The drawing under review shows one solid part. Ordinate dimensions are in mm from its lowest x, y, z. A direction names the side the tool comes from. Round coordinates to 2 decimals unless told otherwise and drop trailing zeros. Write each loop counter-clockwise with the first axis right and the second up, starting at its lowest first coordinate (ties: lowest second). Pieces come first, ordered by that corner, then holes. Notation, with made-up numbers: (-2, 51.5) -> (5, 51.5) arc R20 cw to (5, 72.5) -> close; hole circle Ø8 at (56.25, -12.5). An arc over 180 degrees is marked (long way). Answer in a Markdown table with one row per item. Add a question column.
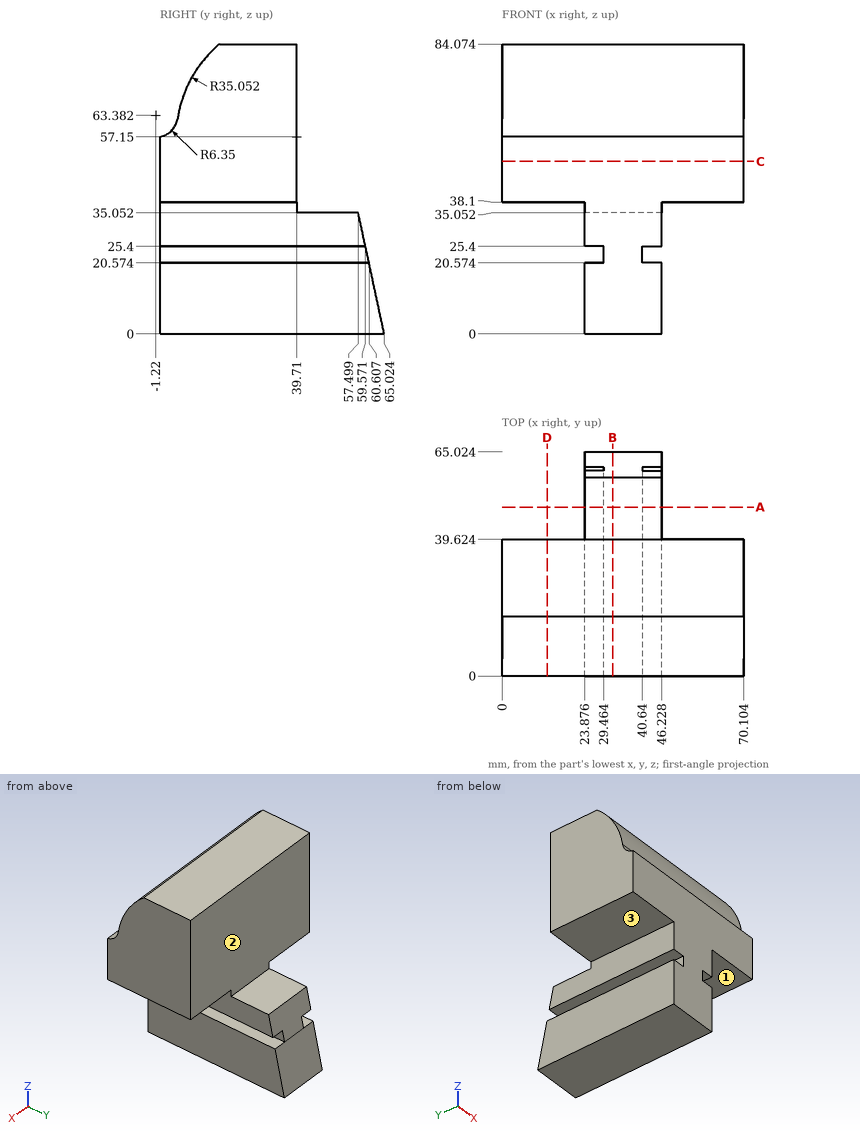
1. Add section C-C on z = 50. Write out the cut boundary in (x, y), plus the area to 3 significant figures.
2. Add section A-A on y = 49. Write out the cut boundary in (x, z).
3. For L1, parallel to Z at x = 41, y = 40.5; L2, parallel to Y at x = 19, z = 56.5; L3, parallel to Z at x = 39.5, y = 56.5, list the stretches that pass through material, from the lowest coordinate up.
4. Add section D-D on x = 13. Write out the cut boundary in (y, z), plus the area to 3 significant figures.
5. Tool access review of the marked faces 1, 2 and 3: name each direction out of +Z, -Z, +X, -X, +Y, -Y from which nothing blocks a thin tool from reaching the whole face with its end or side.
6. Insertion check: pin 1 Ø10.5 at (y, z) = (40, 8) entering from -X; pin 2 Ø5.5 at (x, y) = (39.5, 51) entering from +Z; pin 3 Ø22.5 at (y, z) = (30, 8.5) entering from +X. Each pin has a flat end and moves straight along its axis. Give the tip position at first contact, or say it passes through.
7. Add section B-B on x = 32. Write out the cut boundary in (y, z).
Filled in:
| question | item | result |
|---|---|---|
| 1 | outline | (0, 0) -> (70.1, 0) -> (70.1, 39.62) -> (0, 39.62) -> close |
| 1 | area | 2,780 mm² |
| 2 | outline | (23.88, 0) -> (46.23, 0) -> (46.23, 20.57) -> (40.64, 20.57) -> (40.64, 25.4) -> (46.23, 25.4) -> (46.23, 35.05) -> (23.88, 35.05) -> (23.88, 25.4) -> (29.46, 25.4) -> (29.46, 20.57) -> (23.88, 20.57) -> close |
| 3 | L1 | 0 to 20.57, 25.4 to 35.05 |
| 3 | L2 | 0 to 39.62 |
| 3 | L3 | 0 to 35.05 |
| 4 | outline | (0, 38.1) -> (39.62, 38.1) -> (39.62, 84.07) -> (17.27, 84.07) arc R35.05 ccw to (5.06, 62.43) arc R6.35 cw to (0, 57.15) -> close |
| 4 | area | 1,600 mm² |
| 5 | face 1 | -Z, +X, +Y, -Y |
| 5 | face 2 | +Z, +X, -X, +Y |
| 5 | face 3 | -Z, -X, +Y, -Y |
| 6 | pin 1 | x = 23.88 |
| 6 | pin 2 | z = 35.05 |
| 6 | pin 3 | x = 46.23 |
| 7 | outline | (0, 0) -> (65.02, 0) -> (57.5, 35.05) -> (39.62, 35.05) -> (39.62, 84.07) -> (17.27, 84.07) arc R35.05 ccw to (5.06, 62.43) arc R6.35 cw to (0, 57.15) -> close |
